Part model, mm, in its own coordinate system. Face numbers are marked on the shaded views. A direction names the side the tool comes from. Coordinates: 2 decimals unless noted, no trailing zeros. Write each loop counter-clockwise with the first axis right and the second up, starting at its lowest first coordinate (ties: lowest second). Pieces come first, ordered by that corner, then holes. Notation, with made-up numbers: (55.25, 25.25) -> (101.25, 25.25) arc R26 ccw to (101.25, 63.25) -> close; hole circle Ø8 at (45, 63.25). An arc over 180 degrees is marked (long way). Write item = value, one per line. Start each with the question number.
Q1. Probe line 1 (Y direction, x = 0, z = 0.3); line 2 (X direction, y = 0, z = 0.85); line 3 (Z direction, x = -6.75, y = -3). List the from-to ranges inside material, lowest first.
Q2. Pull direction Y, two halves, no side cores. Call the marked faces 1 and 2: released by +Y, released by -Y, zero draft, split by the parting line, or undercut.
Q3. Band-saw the part on A-A, the plane y = 0. List the corners of the cut face in (x, z).
Q4. Tool access for the marked faces 3 and 4: list every direction of +Z, -Z, +X, -X, +Y, -Y with a clear straight run to the whole face (end or side of a thin tool).
Q5. Band-saw the part on B-B, the plane x = 0. List the corners of the cut face in (y, z), plus the area to 3 significant figures.
Q6. Band-saw the part on C-C, the plane z = 3.55. List the corners of the cut face in (x, y).
Q7. Pin check, flat tips, straight feed: P1, Ø4.5, axis at x = -1, y = -1.5, coming from the +Z side; P2, Ø6.5, axis at x = 0, y = 0, coming from the +Z side; P3, Ø3.5, axis at x = 1.5, y = 1.5, coming from the -Z side. Stop position of each tip, or through.
Q8. Band-saw the part on D-D, the plane y = -15.5. List the corners of the cut face in (x, z).
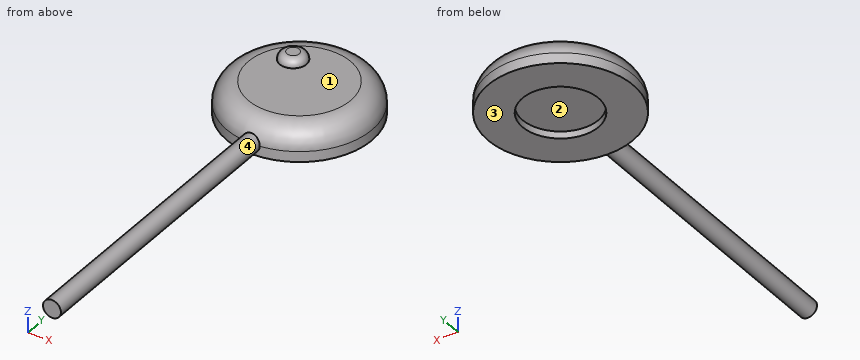
from build123d import *

# Parameters (mm, degrees)
F0_R     = 10.4267
F1_DEPTH = 4.572
F2_R     = 3.066051
F3_R     = 1.288306
F4_DEPTH = 52.578
F5_R     = 1.928538
F6_DEPTH = 1.1176
F7_R     = 1.042457
F8_R     = 5.461
F9_DEPTH = 1.016


with BuildPart() as f1:
    # F0 (on Top) → F1 (new body)
    with BuildSketch(Plane.XY):
        Circle(F0_R)
    extrude(amount=F1_DEPTH)

    # F2
    f2_edges = [f1.edges().sort_by_distance(p)[0] for p in [
        (-10.4267, 0, 4.572),
    ]]
    fillet(f2_edges, radius=F2_R)

    # F3 (on Front) → F4 (join)
    with BuildSketch(Plane.XZ):
        with Locations((0, 1.515293)):
            Circle(F3_R)
    extrude(amount=F4_DEPTH)

    # F5 (on face) → F6 (join)
    with BuildSketch(Plane.XY.offset(4.572)):
        with Locations((-3.190748, 3.358531)):
            Circle(F5_R)
    extrude(amount=F6_DEPTH)

    # F7
    f7_edges = [f1.edges().sort_by_distance(p)[0] for p in [
        (-5.119286, 3.358531, 5.6896),
    ]]
    fillet(f7_edges, radius=F7_R)

    # F8 (on face) → F9 (cut)
    with BuildSketch(Plane(origin=(0, 0, 0), x_dir=(1, 0, 0), z_dir=(0, 0, -1))):
        Circle(F8_R)
    extrude(amount=-F9_DEPTH, mode=Mode.SUBTRACT)


solid = f1.part
Ans:
q1.line_1 = -52.58 to -5.46, 5.46 to 10.43
q1.line_2 = -10.43 to -5.46, 5.46 to 10.43
q1.line_3 = 0 to 4.57
q2.face_1 = zero draft
q2.face_2 = undercut
q3.outline = (-10.43, 0) -> (-5.46, 0) -> (-5.46, 1.02) -> (5.46, 1.02) -> (5.46, 0) -> (10.43, 0) -> (10.43, 1.51) arc R3.07 ccw to (7.36, 4.57) -> (-7.36, 4.57) arc R3.07 ccw to (-10.43, 1.51) -> close
q4.face_3 = -Z, +X, -X, +Y, -Y
q4.face_4 = -Y
q5.outline = (-52.58, 0.23) -> (-10.43, 0.23) -> (-10.43, 0) -> (-5.46, 0) -> (-5.46, 1.02) -> (5.46, 1.02) -> (5.46, 0) -> (10.43, 0) -> (10.43, 1.51) arc R3.07 ccw to (7.36, 4.57) -> (-7.36, 4.57) arc R3.07 ccw to (-10.14, 2.8) -> (-52.58, 2.8) -> close
q5.area = 189 mm2
q6.outline = circle Ø19.29 at (0, 0)
q7.P1 = 4.57
q7.P2 = 5.56
q7.P3 = 1.02
q8.outline = circle Ø2.58 at (0, 1.52)
